Autodesk Inventor part; units mm, degrees
ref_plane "YZ Plane" through (0, 0, 0) normal (1, 0, 0) x (0, 1, 0)
ref_plane "XZ Plane" through (0, 0, 0) normal (0, 1, 0) x (-1, 0, 0)
ref_plane "XY Plane" through (0, 0, 0) normal (0, 0, 1) x (1, 0, 0)
sketch "Sketch3" plane through (0, 0, 0) normal (0, 0, 1) x (1, 0, 0)
  line L0 (-15.7, -16.7) -> (15.7, -16.7)
  line L1 (16.7, -15.7) -> (16.7, 15.7)
  line L2 (15.7, 16.7) -> (-15.7, 16.7)
  line L3 (-16.7, 15.7) -> (-16.7, -15.7)
  line L4 (-16.7, -16.7) -> (16.7, 16.7) construction
  line L5 (16.7, -16.7) -> (-16.7, 16.7) construction
  line L6 (-15.7, 16.7) -> (-16.7, 15.7)
  line L7 (15.7, 16.7) -> (16.7, 15.7)
  line L8 (16.7, -15.7) -> (15.7, -16.7)
  line L9 (-16.7, -15.7) -> (-15.7, -16.7)
  line L10 (-4.9497, -8.8994) -> (4.9497, -8.8994)
  line L11 (4.9497, -8.8994) -> (4.9497, 8.8994)
  line L12 (4.9497, 8.8994) -> (-4.9497, 8.8994)
  line L13 (-4.9497, 8.8994) -> (-4.9497, -8.8994)
  line L14 (-4.9497, -8.8994) -> (4.9497, 8.8994) construction
  line L15 (4.9497, -8.8994) -> (-4.9497, 8.8994) construction
  circle A0 centre (-12.14, 12.625) radius 2.045
  circle A1 centre (12.14, 12.625) radius 2.045
  line L16 (0, -16.7) -> (0, 16.7) construction
  circle A2 centre (-12.14, -12.625) radius 2.045
  circle A3 centre (12.14, -12.625) radius 2.045
  line L17 (12.14, 12.625) -> (-12.14, 12.625) construction
  line L18 (-12.14, 12.625) -> (-12.14, -12.625) construction
  line L19 (-12.14, -12.625) -> (12.14, -12.625) construction
  line L20 (12.14, -12.625) -> (12.14, 12.625) construction
  line L21 (-16.7, 0) -> (16.7, 0) construction
  point P0 (0, 0)
  point P1 (0, 0)
  dimension "d0" = 33.4
  dimension "d1" = 33.4
  dimension "d2" = 1
  dimension "d3" = 1
  dimension "d4" = 1
  dimension "d5" = 1
  dimension "d6" = 1
  dimension "d7" = 1
  dimension "d8" = 1
  dimension "d9" = 1
  dimension "d10" = 9.8994
  dimension "d11" = 17.7988
  dimension "d12" = 4.09
  dimension "d13" = 4.09
  dimension "d17" = 4.09
  dimension "d19" = 24.28
  dimension "d20" = 25.25
  dimension "d21" = 4.09
  dimension "d22" = 12.625
  dimension "d23" = 12.14
extrude "Extrusion1" add sketch "Sketch3" along normal blind 4.1
sketch "Sketch4" plane through (16.7, -15.7, 0) normal (1, 0, 0) x (0, 0, -1)
  circle A0 centre (-2.05, 22.4) radius 1
  circle A1 centre (-2.05, 9) radius 1
  line L0 (0, 32.4) -> (-4.1, 32.4)
  line L1 (0, -1) -> (-4.1, -1)
  line L2 (0, 0) -> (0, 31.4)
  line L3 (-4.1, 31.4) -> (-4.1, 32.4)
  point P0 (0, 15.7)
  dimension "d26" = 2
  dimension "d27" = 10
  dimension "d28" = 10
  dimension "d29" = 13.4
  dimension "d30" = 2.05
  dimension "d31" = 2.05
  dimension "d36" = 2
extrude "Extrusion2" cut sketch "Sketch4" against normal blind 5
sketch "Sketch6" plane through (-16.7, -15.7, 0) normal (-1, 0, 0) x (0, 0, 1)
  circle A0 centre (2.05, 22.4) radius 1
  circle A1 centre (2.05, 22.4) radius 1
  circle A2 centre (2.05, 9) radius 1
  circle A3 centre (2.05, 9) radius 1
  point P0 (0, 15.7)
extrude "Extrusion3" cut sketch "Sketch6" against normal blind 5
thread "Thread1"
thread "Thread2"
thread "Thread3"
thread "Thread4"
equation "\"d3\" = d2"
equation "\"d5\" = d4"
equation "\"d6\" = d4"
equation "\"d7\" = d6"
equation "\"d8\" = d4"
equation "\"d9\" = d8"
properties part number "WG18FLANGEHoled" material "Brass, Soft Yellow"
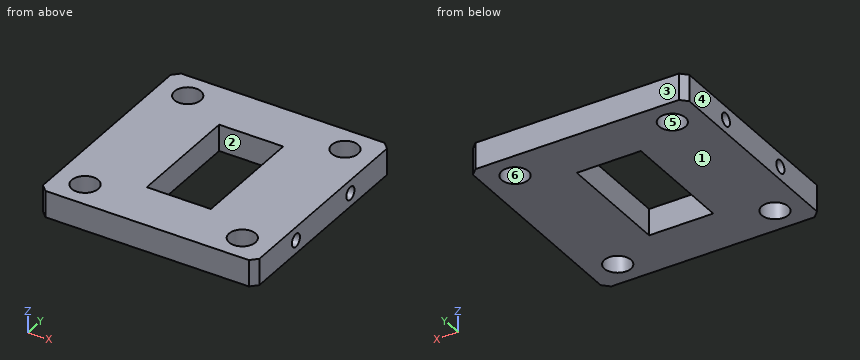
Input: part model. Units: mm. Frame: model coordinates. Face numbers are marked on the shaded views. A direction names the side the tool comes from. Round coordinates to 2 decimals unless told otherwise and drop trailing zeros. Write each loop counter-clockwise with the first axis right and the second up, starting at its lowest first coordinate (ties: lowest second). Pieces come first, ordered by that corner, then holes.
1) Cut plane D-D (z = 3.45). Return the cut outline in (x, y) (3 decimals).
2) Contact query for a flat-ended pin moving along its axis: P1, Ø0.6, axis at y = -6.5, z = 2.5, coming from the -X side. Output: stop coordinate, or through.
3) Cut plane B-B (x = -4). Return the cut outline in (y, z).
4) Ray query, L1, parallel to Y at x = 15.4, z = 2.05; L2, parallel to X at y = -7, z = 1.7; L3, parallel to Y at x = -1, z = 0.85. Return the intervals inside material, ascending.
5) Cut plane C-C (y = -6.7). Return the cut outline in (x, z).
6) Reachability of the marked faces 1 and 2 from +Z, -Z, +X, -X, +Y, -Y: full face, straight path, thin tool, end or side. Return the list, or none.
7) Cut plane A-A (x = -12.14). Return the cut outline in (y, z).
8) Draft query along Y for the marked faces 3, 4, 5 and 6. Return one class per face: pulls with the +Y half, pulls with the -Y half, needs draft (parallel to the pull), parting line crosses it, or undercut.
Geometry says:
1. outline: (-16.7, -15.7) - (-15.7, -16.7) - (15.7, -16.7) - (16.7, -15.7) - (16.7, 15.7) - (15.7, 16.7) - (-15.7, 16.7) - (-16.7, 15.7) - close; hole circle Ø4.09 at (-12.14, -12.625); hole circle Ø4.09 at (-12.14, 12.625); hole (-4.95, -8.899) - (4.95, -8.899) - (4.95, 8.899) - (-4.95, 8.899) - close; hole circle Ø4.09 at (12.14, -12.625); hole circle Ø4.09 at (12.14, 12.625)
2. P1: stops at x = -11.7
3. outline: (-16.7, 0) - (-8.9, 0) - (-8.9, 4.1) - (-16.7, 4.1) - close; (8.9, 0) - (16.7, 0) - (16.7, 4.1) - (8.9, 4.1) - close
4. L1: y = -16.7 to -7.7, -5.7 to 5.7, 7.7 to 16.7
4. L2: x = -11.7 to -4.95, 4.95 to 11.7
4. L3: y = -16.7 to -8.9, 8.9 to 16.7
5. outline: (-16.7, 0) - (-4.95, 0) - (-4.95, 4.1) - (-16.7, 4.1) - (-16.7, 3.05) - (-11.7, 3.05) - (-11.7, 1.05) - (-16.7, 1.05) - close; (4.95, 0) - (16.7, 0) - (16.7, 1.05) - (11.7, 1.05) - (11.7, 3.05) - (16.7, 3.05) - (16.7, 4.1) - (4.95, 4.1) - close
6. face 1: -Z, +X, -X, +Y, -Y
6. face 2: +Z, -Z
7. outline: (-16.7, 0) - (-14.67, 0) - (-14.67, 4.1) - (-16.7, 4.1) - close; (-10.58, 0) - (10.58, 0) - (10.58, 4.1) - (-10.58, 4.1) - close; (14.67, 0) - (16.7, 0) - (16.7, 4.1) - (14.67, 4.1) - close; hole circle Ø2 at (-6.7, 2.05); hole circle Ø2 at (6.7, 2.05)
8. face 3: pulls with the +Y half
8. face 4: needs draft
8. face 5: undercut
8. face 6: undercut
